```python
from build123d import *

# Parameters (mm, degrees)
SKETCH1_W           = 130
SKETCH1_H           = 175
BOSS_EXTRUDE1_DEPTH = 5
CHAMFER1_SIZE       = 5
SKETCH2_W           = 1.5
SKETCH2_H           = 5
BOSS_EXTRUDE2_DEPTH = 5
FILLET2_R           = 1
FILLET3_R           = 1
CUT_EXTRUDE1_DEPTH  = 5


# Some blends are built 0.0001 mm under size
with BuildPart() as part:
    # Sketch1 → Boss-Extrude1 (new body)
    with BuildSketch(Plane(origin=(0, 0, 0), x_dir=(1, 0, 0), z_dir=(0, 1, 0))):
        Rectangle(SKETCH1_W, SKETCH1_H)
    extrude(amount=BOSS_EXTRUDE1_DEPTH)

    # Chamfer1
    chamfer1_edges = [part.edges().sort_by_distance(p)[0] for p in [
        (65, 5, 0),
        (0, 5, -87.5),
        (-65, 5, 0),
        (0, 5, 87.5),
    ]]
    chamfer(chamfer1_edges, length=CHAMFER1_SIZE - 0.0001)  # a hair under: the kernel refuses the full size

    # Sketch2 → Boss-Extrude2 (add)
    with BuildSketch(Plane.XZ):
        Polygon((0, 5), (0, 0), (-1.5, 0), (-1.5, -5), (1.5, -5), (1.5, 5), align=None)
        with Locations((-0.75, 2.5)):
            Rectangle(SKETCH2_W, SKETCH2_H)
    extrude(amount=BOSS_EXTRUDE2_DEPTH)

    # Fillet2
    fillet2_edges = [part.edges().sort_by_distance(p)[0] for p in [
        (-1.5, -5, 0),
        (0, -5, -5),
        (0, -5, 5),
        (1.5, -5, 0),
    ]]
    fillet(fillet2_edges, radius=FILLET2_R)

    # Fillet3
    # the kernel refuses this fillet: 1 mm, written as the material it takes off along each edge
    with BuildSketch(Plane(origin=(-0.5, -4, -4), x_dir=(0, 0, -1), z_dir=(-1, 0, 0))) as fillet3_piece_1_section:
        Polygon((0, 0), (FILLET3_R, 0), (FILLET3_R, FILLET3_R), (0, FILLET3_R), align=None)
    fillet3_piece_1 = extrude(amount=FILLET3_R, mode=Mode.PRIVATE)
    fillet3_piece_1 = fillet3_piece_1 - Plane(origin=(-0.5, -4, -4), x_dir=(0, 0.7071067811865475, 0.7071067811865475), z_dir=(-1, 0, 0)) * Sphere(FILLET3_R, mode=Mode.PRIVATE)
    add(fillet3_piece_1, mode=Mode.SUBTRACT)
    with BuildSketch(Plane(origin=(-0.5, -4, 4), x_dir=(-1, 0, 0), z_dir=(0, 0, 1))) as fillet3_piece_2_section:
        Polygon((0, 0), (FILLET3_R, 0), (FILLET3_R, FILLET3_R), (0, FILLET3_R), align=None)
    fillet3_piece_2 = extrude(amount=FILLET3_R, mode=Mode.PRIVATE)
    fillet3_piece_2 = fillet3_piece_2 - Plane(origin=(-0.5, -4, 4), x_dir=(0.7071067811865475, 0.7071067811865475, 0), z_dir=(0, 0, 1)) * Sphere(FILLET3_R, mode=Mode.PRIVATE)
    add(fillet3_piece_2, mode=Mode.SUBTRACT)
    with BuildSketch(Plane(origin=(0.5, -4, -4), x_dir=(0, 0, -1), z_dir=(1, 0, 0))) as fillet3_piece_3_section:
        Polygon((0, 0), (FILLET3_R, 0), (FILLET3_R, -FILLET3_R), (0, -FILLET3_R), align=None)
    fillet3_piece_3 = extrude(amount=FILLET3_R, mode=Mode.PRIVATE)
    fillet3_piece_3 = fillet3_piece_3 - Plane(origin=(0.5, -4, -4), x_dir=(0, 0.7071067811865475, 0.7071067811865475), z_dir=(1, 0, 0)) * Sphere(FILLET3_R, mode=Mode.PRIVATE)
    add(fillet3_piece_3, mode=Mode.SUBTRACT)
    with BuildSketch(Plane(origin=(0.5, -4, 4), x_dir=(1, 0, 0), z_dir=(0, 0, 1))) as fillet3_piece_4_section:
        Polygon((0, 0), (FILLET3_R, 0), (FILLET3_R, -FILLET3_R), (0, -FILLET3_R), align=None)
    fillet3_piece_4 = extrude(amount=FILLET3_R, mode=Mode.PRIVATE)
    fillet3_piece_4 = fillet3_piece_4 - Plane(origin=(0.5, -4, 4), x_dir=(-0.7071067811865475, 0.7071067811865475, 0), z_dir=(0, 0, 1)) * Sphere(FILLET3_R, mode=Mode.PRIVATE)
    add(fillet3_piece_4, mode=Mode.SUBTRACT)
    with BuildSketch(Plane(origin=(1.5, 0, 5), x_dir=(-1, 0, 0), z_dir=(0, -1, 0)), Plane(origin=(1.5, 0, -5), x_dir=(0, 0, 1), z_dir=(0, -1, 0))) as fillet3_piece_5:
        with BuildLine():
            CenterArc((FILLET3_R, FILLET3_R), FILLET3_R, 180, 90)
            Line((0, FILLET3_R), (0, 0))
            Line((0, 0), (FILLET3_R, 0))
        make_face()
    extrude(amount=4, mode=Mode.SUBTRACT)
    with BuildSketch(Plane(origin=(-1.5, 0, -5), x_dir=(0, 0, 1), z_dir=(0, -1, 0)), Plane(origin=(-1.5, 0, 5), x_dir=(1, 0, 0), z_dir=(0, -1, 0))) as fillet3_piece_6:
        with BuildLine():
            CenterArc((FILLET3_R, -FILLET3_R), FILLET3_R, 90, 90)
            Line((0, -FILLET3_R), (0, 0))
            Line((0, 0), (FILLET3_R, 0))
        make_face()
    extrude(amount=4, mode=Mode.SUBTRACT)

    # Sketch4 → Cut-Extrude1 (cut)
    with BuildSketch(Plane.XZ):
        Polygon((50, -78.775), (26.5, -78.775), (26.5, -8.275), (50, -8.275), (50, -43.75), align=None)
    extrude(amount=-CUT_EXTRUDE1_DEPTH, mode=Mode.SUBTRACT)


solid = part.part
```
Model file for the job. Use its own axes, mm. A direction names the side the tool comes from. Round coordinates to 2 decimals unless told otherwise and drop trailing zeros. Write each loop counter-clockwise with the first axis right and the second up, starting at its lowest first coordinate (ties: lowest second). Pieces come first, ordered by that corner, then holes. Notation, with made-up numbers: M 1.25,89.5 L 54.25,89.5 A9 ccw 54.25,100.5 Z; hole C -25,58.5 d4. An arc over 180 degrees is marked long. Put each result on its own line as item: value.
Item 1: Tool access for faces 1 (the flat face through (38, 2, -78.775)), 2 (the flat face through (62, 3, 1)), 3 (the flat face through (1.5, -2, 0)): list every direction of +Z, -Z, +X, -X, +Y, -Y with a clear straight run to the whole face (end or side of a thin tool).
Responses:
face 1: +Y, -Y
face 2: +Z, -Z, +X, +Y
face 3: +Z, -Z, +X, -Y
Item 2: Mould opens along X. For faces 4 (the flat face through (26.5, 2, -44)), 5 (the flat face through (-15, 0, -1)), 6 (the flat face through (-1.5, -2, 0)) say: +X half, -X half, draft (parallel to the pull), parting line (faces both ways), or undercut.
Responses:
face 4: undercut
face 5: draft
face 6: -X half
Item 3: Flat gauge pins, fed straight in: P1, Ø4, axis at y = 3.5, z = -42, coming from the +X side; P2, Ø6, axis at x = 23.5, y = 3.5, coming from the -Z side; P3, Ø0.8, axis at x = 0, y = -1.5, coming from the -Z side. Where does each tip first touch, or does it go through?
Responses:
P1: x = 63.5
P2: z = -87
P3: z = -5
Item 4: Probe L1, parallel to Y at x = -33, z = 62.5; L2, parallel to Z at x = 17, y = 4.75; L3, parallel to Z at x = 33.5, y = 1 (3 decimals). List the from-to ranges inside material, lowest first. Write a range as from..to.
Responses:
L1: 0..5
L2: -82.75..82.75
L3: -86.5..-78.775, -8.275..86.5
Item 5: Cut at B-B (y = 2). List the corners of the cut face in (x, z) (3 decimals).
Responses:
outline: M -63,-85.5 L 63,-85.5 L 63,85.5 L -63,85.5 Z; hole M 26.5,-78.775 L 50,-78.775 L 50,-8.275 L 26.5,-8.275 Z
